Autodesk Inventor part; units mm, degrees
ref_plane "YZ Plane" through (0, 0, 0) normal (1, 0, 0) x (0, 1, 0)
ref_plane "XZ Plane" through (0, 0, 0) normal (0, 1, 0) x (-1, 0, 0)
ref_plane "XY Plane" through (0, 0, 0) normal (0, 0, 1) x (1, 0, 0)
sketch "Sketch1" plane through (0, 0, 0) normal (0, 0, 1) x (1, 0, 0)
  circle A0 centre (0, 0) radius 11
  circle A1 centre (0, 0) radius 4
  circle A2 centre (0, 0) radius 9.5
  circle A3 centre (0, 0) radius 5.5
  dimension "d0" = 22
  dimension "d1" = 8
  dimension "d2" = 1.5
  dimension "d3" = 1.5
extrude "Extrusion1" add sketch "Sketch1" along normal mid plane 7
extrude "Extrusion2" add sketch "Sketch1" along normal mid plane 6.5 contours A2
chamfer "Chamfer1" distance 0.25 angle 45 8 edges at (-9.5, 0, 3.5) (-11, 0, 3.5) (-4, 0, -3.5) (-5.5, 0, -3.5) (-9.5, 0, -3.5) (-11, 0, -3.5) (-5.5, 0, 3.5) (-4, 0, 3.5)
properties part number "608-2RS Bearing" material "Steel, Carbon"
Geometry: final body of the model. Coordinates: model frame, mm. A direction names the side the tool comes from. Round coordinates to 2 decimals unless told otherwise and drop trailing zeros. Loops run counter-clockwise (first coordinate to the right, second up) from the corner with the lowest first, then second, coordinate; pieces in that order, holes last.
Item 1: Section A-A, the plane z = 0.5. Output: boundary loops of the cut face in (x, y), plus the area to 3 significant figures.
Checked values:
outline: circle Ø22 at (0, 0); hole circle Ø8 at (0, 0)
area: 330 mm2
Item 2: Reachability of faces 1 (the flat face through (4, -4, -3.25)), 2 (the flat face through (2, -4, -3.5)) from +Z, -Z, +X, -X, +Y, -Y: full face, straight path, thin tool, end or side. Return the list, or none.
Checked values:
face 1: -Z
face 2: -Z, +X, -X, +Y, -Y
Item 3: Contact query for flat-ended pins moving along their axis: P1, Ø1.5, axis at x = -1, y = -7, coming from the -Z side; P2, Ø4, axis at x = 7.5, z = 2.5, coming from the -Y side. Output: stop coordinate, or through.
Checked values:
P1: stops at z = -3.25
P2: stops at y = -9.53
Item 4: Line query: L1, parallel to Y at x = 0, z = -3.3; L2, parallel to Y at x = 0, z = 0.5; L3, parallel to Z at x = 6.75, y = 3.75. Output: solid intervals per line, ascending.
Checked values:
L1: y = -10.95 to -9.55, -5.45 to -4.05, 4.05 to 5.45, 9.55 to 10.95
L2: y = -11 to -4, 4 to 11
L3: z = -3.25 to 3.25
Item 5: Mould query, pull axis Y, two halves, no side actions, for faces 3 (the cylindrical face through (-2.38, 10.74, -0.05)), 4 (the flat face through (2, -4, 3.5)), 5 (the flat face through (4, -4, 3.25)). Classes: released by +Y, released by -Y, zero draft, split by the parting line, or undercut.
Checked values:
face 3: split by the parting line
face 4: zero draft
face 5: undercut
